Geometry: final body of the model. Coordinates: model frame, mm. A direction names the side the tool comes from. Coordinates: 2 decimals unless noted, no trailing zeros. Loops run counter-clockwise (first coordinate to the right, second up) from the corner with the lowest first, then second, coordinate; pieces in that order, holes last. Notation, with made-up numbers: (28, 77) - (54, 77) arc R18 cw to (54, 110) - close; hole circle Ø11 at (-32.5, 51). An arc over 180 degrees is marked (long way). Write each question's results on one line, items separated by ' | '. Start each with the question number.
from build123d import *

# Parameters (mm, degrees)
F0_R      = 2.6
F1_DEPTH  = 12.6
F2_R      = 6.1
F3_DEPTH  = 13
F2_R_2    = 8.05
F4_DEPTH  = 6.8
F7_ANGLE  = 180
F10_DEPTH = 13
F11_R     = 1.5


with BuildPart() as f1:
    # F0 (on Top) → F1 (new body)
    with BuildSketch(Plane.XY):
        with BuildLine():
            Line((-27.5, 6), (-29, 6))
            Line((-29, 6), (-29, -6))
            Line((-29, -6), (-27.5, -6))
            ThreePointArc((-27.5, -6), (-26.55, -5.05), (-25.6, -6))
            Line((-25.6, -6), (25.6, -6))
            ThreePointArc((25.6, -6), (26.55, -5.05), (27.5, -6))
            Line((27.5, -6), (29, -6))
            Line((29, -6), (29, 6))
            Line((29, 6), (27.5, 6))
            ThreePointArc((27.5, 6), (26.55, 5.05), (25.6, 6))
            Line((25.6, 6), (-25.6, 6))
            ThreePointArc((-25.6, 6), (-26.55, 5.05), (-27.5, 6))
        make_face()
        with Locations((-23.35, 0)):
            Circle(F0_R, mode=Mode.SUBTRACT)
        with Locations((23.15, 0)):
            Circle(F0_R, mode=Mode.SUBTRACT)
    extrude(amount=F1_DEPTH)

    # F2 (on face) → F3 (cut)
    with BuildSketch(Plane(origin=(0, 6, 0), x_dir=(-1, 0, 0), z_dir=(0, 1, 0))):
        Circle(F2_R)
    extrude(amount=-F3_DEPTH, mode=Mode.SUBTRACT)

    # F2 (on face) → F4 (cut)
    with BuildSketch(Plane(origin=(0, 6, 0), x_dir=(-1, 0, 0), z_dir=(0, 1, 0))):
        Circle(F2_R_2)
        Circle(F2_R, mode=Mode.SUBTRACT)
    extrude(amount=-F4_DEPTH, mode=Mode.SUBTRACT)

    # F9 (on face) → F10 (cut)
    with BuildSketch(Plane(origin=(0, 6, 0), x_dir=(-1, 0, 0), z_dir=(0, 1, 0))):
        with BuildLine():
            Line((-17.3, 7.5), (-10.124722, 7.5))
            ThreePointArc((-10.124722, 7.5), (-5.668333, 11.253), (0, 12.6))
            Line((0, 12.6), (-17.3, 12.6))
            Line((-17.3, 12.6), (-17.3, 7.5))
        make_face()
        with BuildLine():
            ThreePointArc((0, 12.6), (5.668333, 11.253), (10.124722, 7.5))
            Line((10.124722, 7.5), (17.3, 7.5))
            Line((17.3, 7.5), (17.3, 12.6))
            Line((17.3, 12.6), (0, 12.6))
        make_face()
    extrude(amount=-F10_DEPTH, mode=Mode.SUBTRACT)

    # F11
    f11_edges = [f1.edges().sort_by_distance(p)[0] for p in [
        (17.3, 0, 7.5),
        (10.124722, 0, 7.5),
        (-10.124722, 0, 7.5),
        (-17.3, 0, 7.5),
    ]]
    fillet(f11_edges, radius=F11_R)


with BuildPart() as f5_1:
    # F5: copy of F1
    add(f1.part)


with BuildPart() as f7_1:
    # F7: copy of F1
    add(f1.part.rotate(Axis((0, 1.422519, 0), (0, 1, 0)), F7_ANGLE))


solid = f1.part
1) Access query for faces 1 (the flat face through (0, -0.8, 6.4)), 2 (the cylindrical face through (26.57, 5.05, 6.21)), 3 (the flat face through (-13, 0, 7.5)). Directions: +Z, -Z, +X, -X, +Y, -Y. A direction counts if a zero-diameter tool reaches every point of the face in a straight line with its end or side. Return the directions, or none.
2) Section query B-B on x = -23.35. Output: boundary loops of the cut face in (y, z).
3) Section query C-C on z = 9.5. Output: boundary loops of the cut face in (x, y).
4) Material intervals for line 1 (Y direction, x = -23.35, z = 6.5); line 2 (X direction, y = -3.75, z = 11.25); line 3 (X direction, y = -0.75, z = 1.25), sorted ascending. Write a range as [from, to].
5) Section query A-A on z = 3. Output: boundary loops of the cut face in (x, y), and give its area (3 significant figures).
6) Pull-direction query (X, two-part tool) for faces 4 (the flat face through (20, 0, 12.6)), 5 (the flat face through (-29, 0, 6)), 6 (the cylindrical face through (-10.22, -0.08, 7.64)); classes: released by +X, released by -X, zero draft, split by the parting line, or undercut.
7) Pin query (flat end, axial travel): pin 1 Ø2.5 at (x, y) = (-14, 1.5) entering from +Z; pin 2 Ø4.5 at (x, y) = (-23.35, 0) entering from -Z; pin 3 Ø2 at (x, y) = (-7.5, -2.5) entering from +Z; pin 4 Ø4 at (x, z) = (-2, 4) entering from +Y. Return the tip coordinate at first contact, or that it passes through.
8) Section query D-D on x = 26.55. Output: boundary loops of the cut face in (y, z).
Returned:
1) face 1: -Z, +Y | face 2: +Z, -Z, +Y | face 3: +Z, +Y, -Y
2) outline: (-6, 0) - (-2.6, 0) - (-2.6, 12.6) - (-6, 12.6) - close; (2.6, 0) - (6, 0) - (6, 12.6) - (2.6, 12.6) - close
3) outline: (-29, -6) - (-27.5, -6) arc R0.95 cw to (-25.6, -6) - (-17.3, -6) - (-17.3, 6) - (-25.6, 6) arc R0.95 cw to (-27.5, 6) - (-29, 6) - close; (-8.28, -6) - (8.28, -6) - (8.28, 6) - (-8.28, 6) - close; (17.3, -6) - (25.6, -6) arc R0.95 cw to (27.5, -6) - (29, -6) - (29, 6) - (27.5, 6) arc R0.95 cw to (25.6, 6) - (17.3, 6) - close; hole circle Ø5.2 at (-23.35, 0); hole circle Ø5.2 at (23.15, 0)
4) line 1: y = [-6, -2.6], [2.6, 6] | line 2: x = [-29, -17.3], [-5.67, 5.67], [17.3, 29] | line 3: x = [-29, -25.84], [-20.86, -7.95], [7.95, 20.66], [25.64, 29]
5) outline: (-29, -6) - (-27.5, -6) arc R0.95 cw to (-25.6, -6) - (-5.31, -6) - (-5.31, -0.8) - (-7.47, -0.8) - (-7.47, 6) - (-25.6, 6) arc R0.95 cw to (-27.5, 6) - (-29, 6) - close; (5.31, -6) - (25.6, -6) arc R0.95 cw to (27.5, -6) - (29, -6) - (29, 6) - (27.5, 6) arc R0.95 cw to (25.6, 6) - (7.47, 6) - (7.47, -0.8) - (5.31, -0.8) - close; hole circle Ø5.2 at (-23.35, 0); hole circle Ø5.2 at (23.15, 0) | area: 491 mm²
6) face 4: zero draft | face 5: released by -X | face 6: undercut
7) pin 1: stops at z = 7.5 | pin 2: passes through | pin 3: stops at z = 10.79 | pin 4: stops at y = -0.8
8) outline: (-5.05, 0) - (5.05, 0) - (5.05, 12.6) - (-5.05, 12.6) - close
